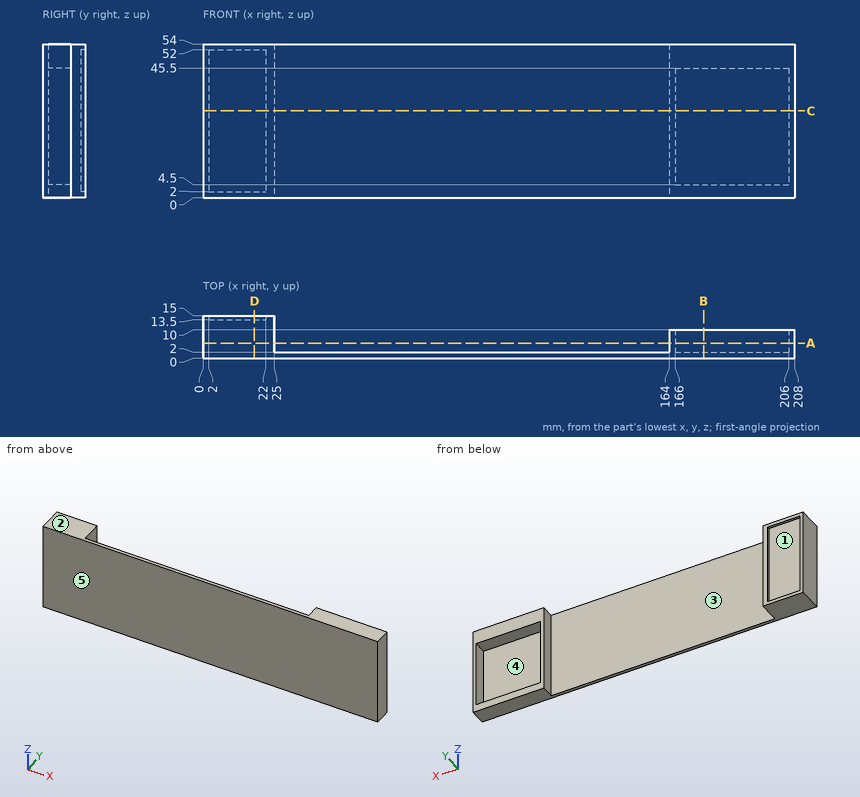
Job drawing, mm, ordinate dimensions from the low corner. One solid piece. A direction names the side the tool comes from. Give positions to 0.01 mm unless a question says otherwise; leave off trailing zeros. Loops run counter-clockwise (first coordinate to the right, second up) from the corner with the lowest first, then second, coordinate; pieces in that order, holes last. Notation, with made-up numbers: (-17, 3.25) - (-2, 3.25) arc R36 ccw to (-2, 42.25) - close; hole circle Ø8 at (0, -27.75). An arc over 180 degrees is marked (long way). Use one line per item in the form item = value.
(1) Drop flat-ended pins along their axis: P1, Ø1, axis at y = 13, z = 26.5, coming from the +X side; P2, Ø6, axis at x = 182.5, z = 40.5, coming from the +Y side. Give the stop position or say it passes through.
Determined:
P1 = 25
P2 = 2
(2) Cut at B-B (x = 176). Give the cut face in (y, z), then the cut area to 3 significant figures.
Determined:
outline = (0, 0) - (10, 0) - (10, 4.5) - (2, 4.5) - (2, 45.5) - (10, 45.5) - (10, 54) - (0, 54) - close
area = 212 mm^2
(3) Drill centre lines: L1, parallel to X at y = 4.5, z = 24; L2, parallel to Z at x = 199, y = 9.5; L3, parallel to Y at x = 133, z = 6.5. Where is each one in solid material? Low to high.
Determined:
L1 = 0 to 25, 164 to 166, 206 to 208
L2 = 0 to 4.5, 45.5 to 54
L3 = 0 to 2
(4) Cut at A-A (y = 5.25). Give the cut face in (x, z), then the cut area to 3 significant figures.
Determined:
outline = (0, 0) - (25, 0) - (25, 54) - (0, 54) - close; (164, 0) - (208, 0) - (208, 54) - (164, 54) - close; hole (166, 4.5) - (206, 4.5) - (206, 45.5) - (166, 45.5) - close
area = 2,090 mm^2
(5) Cut at C-C (z = 30.5). Give the cut face in (x, y).
Determined:
outline = (0, 0) - (208, 0) - (208, 10) - (206, 10) - (206, 2) - (166, 2) - (166, 10) - (164, 10) - (164, 2) - (25, 2) - (25, 15) - (22, 15) - (22, 13.5) - (2, 13.5) - (2, 15) - (0, 15) - close
(6) 3-axis set-ups, long thin cutter, end or side, ignore diameter. For the marked faces 1, 2 and 3: which of +Z, -Z, +X, -X, +Y, -Y reach the whole face in a straight line?
Determined:
face_1 = +Y
face_2 = +Z, +X, -X, +Y, -Y
face_3 = +Z, -Z, +Y
(7) Pull direction X, two halves, no side cores. Call the marked faces 4 and 5: pulls with the +X half, pulls with the -X half, needs draft (parallel to the pull), parting line crosses it, or undercut.
Determined:
face_4 = undercut
face_5 = needs draft
(8) Cut at D-D (x = 18). Give the cut face in (y, z), then the cut area to 3 significant figures.
Determined:
outline = (0, 0) - (15, 0) - (15, 2) - (13.5, 2) - (13.5, 52) - (15, 52) - (15, 54) - (0, 54) - close
area = 735 mm^2
